from build123d import *

# Parameters (mm, degrees)
BOSS_EXTRUDE1_DEPTH = 70
SKETCH3_W           = 50
SKETCH3_H           = 66
CUT_EXTRUDE1_DEPTH  = 88.388879183
SKETCH4_R           = 11
CUT_EXTRUDE2_DEPTH  = 10
SKETCH5_R           = 6
CUT_EXTRUDE3_DEPTH  = 10


with BuildPart() as part:
    # Sketch1 → Boss-Extrude1 (new body)
    with BuildSketch(Plane.XY):
        Polygon((-17.141906192, 0), (32.858093808, 0), (32.858093808, 10), (42.858093808, 10), (42.858093808, -30), (32.858093808, -30), (32.858093808, -20), (-17.141906192, -20), (-17.141906192, -30), (-27.141906192, -30), (-27.141906192, 10), (-17.141906192, 10), align=None)
    extrude(amount=BOSS_EXTRUDE1_DEPTH)

    # Sketch3 → Cut-Extrude1 (cut, through all)
    with BuildSketch(Plane(origin=(0, 0, 0), x_dir=(1, 0, 0), z_dir=(0, 1, 0))):
        with Locations((7.858093808, -35)):
            Rectangle(SKETCH3_W, SKETCH3_H)
    extrude(amount=-CUT_EXTRUDE1_DEPTH, mode=Mode.SUBTRACT)

    # Sketch4 → Cut-Extrude2 (cut)
    with BuildSketch(Plane(origin=(42.858093808, 0, 0), x_dir=(0, 0, -1), z_dir=(1, 0, 0))):
        with Locations((-35, -10)):
            Circle(SKETCH4_R)
    extrude(amount=-CUT_EXTRUDE2_DEPTH, mode=Mode.SUBTRACT)

    # Sketch5 → Cut-Extrude3 (cut)
    with BuildSketch(Plane(origin=(42.858093808, 0, 0), x_dir=(0, 0, -1), z_dir=(1, 0, 0))):
        with Locations((-13, -10)):
            Circle(SKETCH5_R)
        with Locations((-57, -10)):
            Circle(SKETCH5_R)
    extrude(amount=-CUT_EXTRUDE3_DEPTH, mode=Mode.SUBTRACT)


solid = part.part
Can you work these out from the model? Positions are in its coordinate system, mm. A direction names the side the tool comes from. Round coordinates to 2 decimals unless told otherwise and drop trailing zeros. Loops run counter-clockwise (first coordinate to the right, second up) from the corner with the lowest first, then second, coordinate; pieces in that order, holes last. Notation, with made-up numbers: (59.5, 11.25) - (109.5, 11.25) arc R23 ccw to (109.5, 33.25) - close; hole circle Ø5 at (76, 49). An arc over 180 degrees is marked (long way). Write item = value, one per line. Start each with the question number.
(1) For P1, Ø1, axis at x = 3.5, z = 69.5, coming from the +Y side; P2, Ø1.6, axis at x = 0.5, z = 1, coming from the -Y side; P3, Ø11, axis at y = -10, z = 57, coming from the +X side, each with a flat end and sliding along its axis, tell me the tip position at first contact or that it passes through.
(2) For faces 1 (the face through (38, -10, 63)), 2 (the face through (8, -20, 69)), 3 (the face through (8, 0, 1)), 4 (the face through (8, -10, 68)), which set-ups out of +Z, -Z, +X, -X, +Y, -Y let a thin tool reach every point of the face, with its end or its side?
(3) If we section it at B-B (x = 7): Please give me the cut outline in (y, z), and give its area (3 significant figures).
(4) If we section it at C-C (y = -10): Please give me the cut outline in (x, z), and give its area (3 significant figures).
(5) If we mould it in two halves opening along Z, with no side actions, what happens to faces 5 (the face through (8, -10, 70)), 6 (the face through (-17.142, -10, 35)), 7 (the face through (38, -30, 35))? For each: released by +Z, released by -Z, zero draft, split by the parting line, or undercut.
(6) If I drill on probe 1 along X at (y, z) = (-5.5, 3); probe 2 along Y at (x, z) = (38.5, 35); probe 3 along Y at (x, z) = (38.25, 13), over which ranges is the centre line in solid material (lowest first)? Write a range as [from, to].
(7) If we section it at A-A (z = 13): Please give me the cut outline in (x, y), and give its area (3 significant figures).
(8) If we section it at D-D (z = 23): Please give me the cut outline in (x, y), and give its area (3 significant figures).
Ans:
q1.P1 = 0
q1.P2 = -20
q1.P3 = -17.14
q2.face_1 = +X
q2.face_2 = +Z, -Z, -Y
q2.face_3 = +Z, -Z, +Y
q2.face_4 = +Y, -Y
q3.outline = (-20, 0) - (0, 0) - (0, 2) - (-20, 2) - close; (-20, 68) - (0, 68) - (0, 70) - (-20, 70) - close
q3.area = 80.0 mm²
q4.outline = (-27.14, 0) - (42.86, 0) - (42.86, 7) - (32.86, 7) - (32.86, 2) - (-17.14, 2) - (-17.14, 68) - (32.86, 68) - (32.86, 63) - (42.86, 63) - (42.86, 70) - (-27.14, 70) - close; (32.86, 19) - (42.86, 19) - (42.86, 24) - (32.86, 24) - close; (32.86, 46) - (42.86, 46) - (42.86, 51) - (32.86, 51) - close
q4.area = 1,140 mm²
q5.face_5 = released by +Z
q5.face_6 = undercut
q5.face_7 = zero draft
q6.probe_1 = [-27.14, -17.14], [32.86, 42.86]
q6.probe_2 = [-30, -21], [1, 10]
q6.probe_3 = [-30, -16], [-4, 10]
q7.outline = (-27.14, -30) - (-17.14, -30) - (-17.14, 10) - (-27.14, 10) - close; (32.86, -30) - (42.86, -30) - (42.86, -16) - (32.86, -16) - close; (32.86, -4) - (42.86, -4) - (42.86, 10) - (32.86, 10) - close
q7.area = 680 mm²
q8.outline = (-27.14, -30) - (-17.14, -30) - (-17.14, 10) - (-27.14, 10) - close; (32.86, -30) - (42.86, -30) - (42.86, 10) - (32.86, 10) - close
q8.area = 800 mm²
